from build123d import *

# Parameters (mm, degrees)
SKETCH1_W          = 153.56078
SKETCH1_H          = 114.3
SKETCH1_R          = 2.413
BASE_FLANGE1_DEPTH = 2.38125
FILLET1_R          = 6.35
SKETCH7_W          = 19.05
SKETCH7_H          = 114.3
CUT_EXTRUDE2_DEPTH = 2.54
FILLET2_R          = 6.35
FILLET3_R          = 6.35


# Sheet-metal steps are written as plain solids
with BuildPart() as part:
    # Sketch1 → Base-Flange1 (new body)
    with BuildSketch(Plane(origin=(0, 0, 0), x_dir=(1, 0, 0), z_dir=(0, 1, 0))):
        Rectangle(SKETCH1_W, SKETCH1_H)
        with Locations(Location((-63.5, -51.59375, 0), (0, 0, 270))):
            Circle(SKETCH1_R, mode=Mode.SUBTRACT)
        with Locations(Location((-38.1, -51.59375, 0), (0, 0, 270))):
            Circle(SKETCH1_R, mode=Mode.SUBTRACT)
        with Locations(Location((-12.7, -51.59375, 0), (0, 0, 270))):
            Circle(SKETCH1_R, mode=Mode.SUBTRACT)
        with Locations(Location((12.7, -51.59375, 0), (0, 0, 270))):
            Circle(SKETCH1_R, mode=Mode.SUBTRACT)
        with Locations(Location((38.1, -51.59375, 0), (0, 0, 270))):
            Circle(SKETCH1_R, mode=Mode.SUBTRACT)
        with Locations(Location((63.5, -51.59375, 0), (0, 0, 270))):
            Circle(SKETCH1_R, mode=Mode.SUBTRACT)
        with Locations(Location((63.5, 51.59375, 0), (0, 0, 270))):
            Circle(SKETCH1_R, mode=Mode.SUBTRACT)
        with Locations(Location((38.1, 51.59375, 0), (0, 0, 270))):
            Circle(SKETCH1_R, mode=Mode.SUBTRACT)
        with Locations(Location((12.7, 51.59375, 0), (0, 0, 270))):
            Circle(SKETCH1_R, mode=Mode.SUBTRACT)
        with Locations(Location((-12.7, 51.59375, 0), (0, 0, 270))):
            Circle(SKETCH1_R, mode=Mode.SUBTRACT)
        with Locations(Location((-38.1, 51.59375, 0), (0, 0, 270))):
            Circle(SKETCH1_R, mode=Mode.SUBTRACT)
        with Locations(Location((-63.5, 51.59375, 0), (0, 0, 270))):
            Circle(SKETCH1_R, mode=Mode.SUBTRACT)
        Polygon((60.90539, -41.275), (-63.104482091, -41.275), (-63.104482091, 41.275), (21.327886111, 41.275), (60.90539, 41.275), (60.90539, 15.875), align=None, mode=Mode.SUBTRACT)
    extrude(amount=-BASE_FLANGE1_DEPTH)

    # Fillet1
    fillet1_edges = [part.edges().sort_by_distance(p)[0] for p in [
        (-76.78039, -1.190625, -57.15),
        (76.78039, -1.190625, -57.15),
        (76.78039, -1.190625, 57.15),
        (-76.78039, -1.190625, 57.15),
    ]]
    fillet(fillet1_edges, radius=FILLET1_R)

    # Sketch7 → Cut-Extrude2 (cut)
    with BuildSketch(Plane(origin=(0, -2.38125, 0), x_dir=(-1, 0, 0), z_dir=(0, -1, 0))):
        with Locations((67.25539, 0)):
            Rectangle(SKETCH7_W, SKETCH7_H)
    extrude(amount=-CUT_EXTRUDE2_DEPTH, mode=Mode.SUBTRACT)

    # Fillet2
    fillet2_edges = [part.edges().sort_by_distance(p)[0] for p in [
        (-57.73039, -1.190625, 41.275),
        (-57.73039, -1.190625, -41.275),
        (-57.73039, -1.190625, 57.15),
        (-57.73039, -1.190625, -57.15),
    ]]
    fillet(fillet2_edges, radius=FILLET2_R)

    # Fillet3
    fillet3_edges = [part.edges().sort_by_distance(p)[0] for p in [
        (60.90539, -1.190625, -41.275),
        (60.90539, -1.190625, 41.275),
    ]]
    fillet(fillet3_edges, radius=FILLET3_R)


solid = part.part
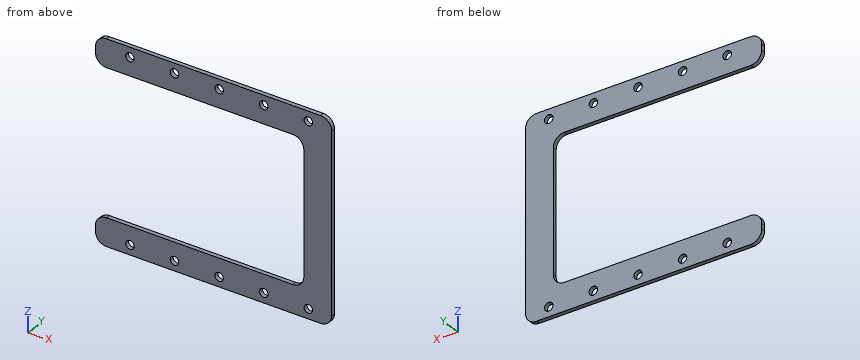
Model file for the job. Use its own axes, mm. Give positions to 0.01 mm unless a question says otherwise; leave off trailing zeros. Order: outer loops, then holes, each group sorted by start corner. A loop starts at its lowest first (then second) coordinate and runs counter-clockwise, first axis right, second up. Notation, with made-up numbers: M 68.5,-36.5 L 90.5,-36.5 A11 cw 90.5,-32.5 Z; hole C -28,-3.75 d1. An arc over 180 degrees is marked long. Put each result on its own line as item: value. Start each with the question number.
(1) Drill centre lines: L1, parallel to Z at x = -20, y = -1.85 (3 decimals); L2, parallel to X at y = -1.2, z = -15; L3, parallel to X at y = -1.25, z = 47.5. Where is each one in solid material? Low to high. Write a range as [from, to].
(2) Band-saw the part on D-D on z = 18.5. Give the cut face in (x, y).
(3) Band-saw the part on B-B on y = -1.5. Count the separate pieces of the cut face and the enclosed holes in it, then the cut area to 3 significant figures.
(4) Band-saw the part on C-C on x = 63.5. Give the cut face in (y, z), then the cut area to 3 significant figures.
(5) Band-saw the part on A-A on x = 0. Give the cut face in (y, z) (3 decimals).
(6) Pin check, flat tip, straight feed: pin 1 Ø0.7 at (y, z) = (-1, 7) entering from -X. Stop position of the tip, or through.
Results below:
1. L1: z = [-57.15, -41.275], [41.275, 57.15]
1. L2: x = [60.91, 76.78]
1. L3: x = [-57.73, 76.78]
2. outline: M 60.91,-2.38 L 76.78,-2.38 L 76.78,0 L 60.91,0 Z
3. separate pieces: 1
3. enclosed holes: 10
3. area: 5,360 mm2
4. outline: M -2.38,-57.15 L 0,-57.15 L 0,-54.01 L -2.38,-54.01 Z; M -2.38,-49.18 L 0,-49.18 L 0,49.18 L -2.38,49.18 Z; M -2.38,54.01 L 0,54.01 L 0,57.15 L -2.38,57.15 Z
4. area: 249 mm2
5. outline: M -2.381,-57.15 L 0,-57.15 L 0,-41.275 L -2.381,-41.275 Z; M -2.381,41.275 L 0,41.275 L 0,57.15 L -2.381,57.15 Z
6. pin 1: stops at x = 60.91
